Could you check a few things on this model? Use its own coordinates, in mm. A direction names the side the tool comes from. Give positions to 0.01 mm unless a question says otherwise; leave off trailing zeros. Write each loop counter-clockwise with the first axis right and the second up, starting at its lowest first coordinate (ties: lowest second). Pieces come first, ordered by that corner, then holes. Notation, with made-up numbers: M 31.25,57.5 L 60.25,57.5 A25 cw 60.25,80.5 Z; hole C 78,82.25 d2. An arc over 180 degrees is marked long. Use one line per item in the form item = value.
from build123d import *

# Parameters (mm, degrees)
SKETCH1_W           = 38
SKETCH1_H           = 29
BOSS_EXTRUDE1_DEPTH = 50
SKETCH2_W           = 13
SKETCH2_H           = 29
BOSS_EXTRUDE2_DEPTH = 40
CHAMFER1_SIZE       = 40
SKETCH3_W           = 10
SKETCH3_H           = 29
CUT_EXTRUDE1_DEPTH  = 14
FILLET1_R           = 12


with BuildPart() as part:
    # Sketch1 → Boss-Extrude1 (new body)
    with BuildSketch(Plane.XY):
        with Locations((-19, 0)):
            Rectangle(SKETCH1_W, SKETCH1_H)
    extrude(amount=-BOSS_EXTRUDE1_DEPTH)

    # Sketch2 → Boss-Extrude2 (add)
    with BuildSketch(Plane(origin=(0, 0, -50), x_dir=(-1, 0, 0), z_dir=(0, 0, -1))):
        with Locations((6.5, 0)):
            Rectangle(SKETCH2_W, SKETCH2_H)
    extrude(amount=BOSS_EXTRUDE2_DEPTH)

    # Chamfer1
    # the kernel refuses this chamfer: 40 mm, written as the material it takes off along each edge
    with BuildSketch(Plane(origin=(-38, -117.367319519, -50), x_dir=(-0.027495876610586317, 0, 0.9996219169112968), z_dir=(0, 1, 0))) as chamfer1_piece_1_section:
        Polygon((CHAMFER1_SIZE * 0.999621916911, CHAMFER1_SIZE * 0.0274958766106), (-CHAMFER1_SIZE * 0.0274958766106, CHAMFER1_SIZE * 0.999621916911), (0, 0), align=None)
    chamfer1_piece_1 = extrude(amount=234.734639037, mode=Mode.PRIVATE)
    chamfer1_piece_1 = split(chamfer1_piece_1, bisect_by=Plane(origin=(-13, 0, -35.169417803), z_dir=(-1, 0, 0)), keep=Keep.TOP, mode=Mode.PRIVATE)
    add(chamfer1_piece_1, mode=Mode.SUBTRACT)

    # Sketch3 → Cut-Extrude1 (cut)
    with BuildSketch(Plane(origin=(0, 0, -90), x_dir=(-1, 0, 0), z_dir=(0, 0, -1))):
        with Locations((8, 0)):
            Rectangle(SKETCH3_W, SKETCH3_H)
    extrude(amount=-CUT_EXTRUDE1_DEPTH, mode=Mode.SUBTRACT)

    # Fillet1
    fillet1_edges = [part.edges().sort_by_distance(p)[0] for p in [
        (-1.5, -14.5, -90),
        (-1.5, 14.5, -90),
    ]]
    fillet(fillet1_edges, radius=FILLET1_R)


solid = part.part
1) I want a section at A-A, the plane y = 0.25. Please give me the cut outline in (x, z).
Checked values:
outline = M -38,-10 L -13,-35 L -13,-76 L -3,-76 L -3,-90 L 0,-90 L 0,0 L -38,0 Z
2) I want a section at C-C, the plane x = -35. Please give me the cut outline in (y, z).
Checked values:
outline = M -14.5,-13 L 14.5,-13 L 14.5,0 L -14.5,0 Z
3) If I drill on L1, parallel to X at y = -6, z = -13; L2, parallel to X at y = 3, z = -83.5; L3, parallel to Z at x = -4, y = 5.25, over which ranges is the centre line in solid material (lowest first)?
Checked values:
L1 = -35 to 0
L2 = -3 to 0
L3 = -76 to 0
4) For pin 1 Ø1.5 at (x, y) = (-5, 3) entering from -Z; pin 2 Ø5 at (x, y) = (-26, -9.5) entering from -Z; pin 3 Ø14.5 at (y, z) = (4, -55.5) entering from -X, each with a flat end and sliding along its axis, tell me the tip position at first contact or that it passes through.
Checked values:
pin_1 = -76
pin_2 = -24.5
pin_3 = -13
5) I want a section at B-B, the plane z = -30. Please give me the cut outline in (x, y).
Checked values:
outline = M -18,-14.5 L 0,-14.5 L 0,14.5 L -18,14.5 Z
6) I want a section at D-D, the plane y = -8.5. Please give me the cut outline in (x, z), plus the area to 3 significant figures.
Checked values:
outline = M -38,-10 L -13,-35 L -13,-76 L -3,-76 L -3,-88.39 L 0,-88.39 L 0,0 L -38,0 Z
area = 1,590 mm2
7) For faces 1 (the cylindrical face through (-1.52, -10.89, -86.58)), 2 (the flat face through (-13, 0, -55)), which set-ups out of +Z, -Z, +X, -X, +Y, -Y let a thin tool reach every point of the face, with its end or its side?
Checked values:
face_1 = -Z, +X, -X, -Y
face_2 = -Z, -X, +Y, -Y
